from build123d import *

# Parameters (mm, degrees)
MODEL_R         = 24.25
MODEL_R_2       = 2
EXTRUDE_1_DEPTH = 2


with BuildPart() as part:
    # Model → 凸台-拉伸1 (new body)
    with BuildSketch(Plane.XY):
        with Locations((1461.027973693, 726.314415121)):
            Circle(MODEL_R)
        with Locations((1461.027973693, 726.314415121)):
            Circle(MODEL_R_2, mode=Mode.SUBTRACT)
        with BuildLine():
            ThreePointArc((1454.730507071, 746.347934885), (1450.527973693, 744.5009486), (1446.827169961, 741.784941077))
            ThreePointArc((1446.827169961, 741.784941077), (1445.858696219, 739.705372638), (1446.642743938, 737.549493362))
            ThreePointArc((1446.642743938, 737.549493362), (1449.919857233, 734.687570493), (1453.749968469, 732.623515752))
            ThreePointArc((1453.749968469, 732.623515752), (1457.242892618, 732.870367853), (1459.203134883, 735.771902849))
            ThreePointArc((1459.203134883, 735.771902849), (1459.33066666, 740.120903849), (1458.490725399, 744.389928648))
            ThreePointArc((1458.490725399, 744.389928648), (1457.015703038, 746.146873529), (1454.730507071, 746.347934885))
        make_face(mode=Mode.SUBTRACT)
        with BuildLine():
            ThreePointArc((1440.529703339, 730.877408929), (1440.027973693, 726.314415121), (1440.529703339, 721.751421313))
            ThreePointArc((1440.529703339, 721.751421313), (1441.846425564, 719.87291423), (1444.105495645, 719.473979835))
            ThreePointArc((1444.105495645, 719.473979835), (1448.222550201, 720.881081765), (1451.925129659, 723.166028024))
            ThreePointArc((1451.925129659, 723.166028024), (1453.457811542, 726.314415121), (1451.925129659, 729.462802217))
            ThreePointArc((1451.925129659, 729.462802217), (1448.222550201, 731.747748477), (1444.105495645, 733.154850407))
            ThreePointArc((1444.105495645, 733.154850407), (1441.846425564, 732.755916011), (1440.529703339, 730.877408929))
        make_face(mode=Mode.SUBTRACT)
        with BuildLine():
            ThreePointArc((1446.827169961, 710.843889164), (1450.527973693, 708.127881641), (1454.730507071, 706.280895356))
            ThreePointArc((1454.730507071, 706.280895356), (1457.015703038, 706.481956712), (1458.490725399, 708.238901593))
            ThreePointArc((1458.490725399, 708.238901593), (1459.33066666, 712.507926392), (1459.203134883, 716.856927392))
            ThreePointArc((1459.203134883, 716.856927392), (1457.242892618, 719.758462388), (1453.749968469, 720.005314489))
            ThreePointArc((1453.749968469, 720.005314489), (1449.919857233, 717.941259748), (1446.642743938, 715.079336879))
            ThreePointArc((1446.642743938, 715.079336879), (1445.858696219, 712.923457603), (1446.827169961, 710.843889164))
        make_face(mode=Mode.SUBTRACT)
        with BuildLine():
            ThreePointArc((1467.325440315, 706.280895356), (1471.527973693, 708.127881641), (1475.228777425, 710.843889164))
            ThreePointArc((1475.228777425, 710.843889164), (1476.197251167, 712.923457603), (1475.413203447, 715.079336879))
            ThreePointArc((1475.413203447, 715.079336879), (1472.136090152, 717.941259748), (1468.305978916, 720.005314489))
            ThreePointArc((1468.305978916, 720.005314489), (1464.813054768, 719.758462388), (1462.852812503, 716.856927392))
            ThreePointArc((1462.852812503, 716.856927392), (1462.725280725, 712.507926392), (1463.565221986, 708.238901593))
            ThreePointArc((1463.565221986, 708.238901593), (1465.040244347, 706.481956712), (1467.325440315, 706.280895356))
        make_face(mode=Mode.SUBTRACT)
        with BuildLine():
            ThreePointArc((1481.526244047, 721.751421313), (1482.027973693, 726.314415121), (1481.526244047, 730.877408929))
            ThreePointArc((1481.526244047, 730.877408929), (1480.209521821, 732.755916011), (1477.950451741, 733.154850407))
            ThreePointArc((1477.950451741, 733.154850407), (1473.833397185, 731.747748477), (1470.130817726, 729.462802217))
            ThreePointArc((1470.130817726, 729.462802217), (1468.598135843, 726.314415121), (1470.130817726, 723.166028024))
            ThreePointArc((1470.130817726, 723.166028024), (1473.833397185, 720.881081765), (1477.950451741, 719.473979835))
            ThreePointArc((1477.950451741, 719.473979835), (1480.209521821, 719.87291423), (1481.526244047, 721.751421313))
        make_face(mode=Mode.SUBTRACT)
        with BuildLine():
            ThreePointArc((1475.228777425, 741.784941077), (1471.527973693, 744.5009486), (1467.325440315, 746.347934885))
            ThreePointArc((1467.325440315, 746.347934885), (1465.040244347, 746.146873529), (1463.565221986, 744.389928648))
            ThreePointArc((1463.565221986, 744.389928648), (1462.725280725, 740.120903849), (1462.852812503, 735.771902849))
            ThreePointArc((1462.852812503, 735.771902849), (1464.813054768, 732.870367853), (1468.305978916, 732.623515752))
            ThreePointArc((1468.305978916, 732.623515752), (1472.136090152, 734.687570493), (1475.413203447, 737.549493362))
            ThreePointArc((1475.413203447, 737.549493362), (1476.197251167, 739.705372638), (1475.228777425, 741.784941077))
        make_face(mode=Mode.SUBTRACT)
    extrude(amount=EXTRUDE_1_DEPTH)


solid = part.part
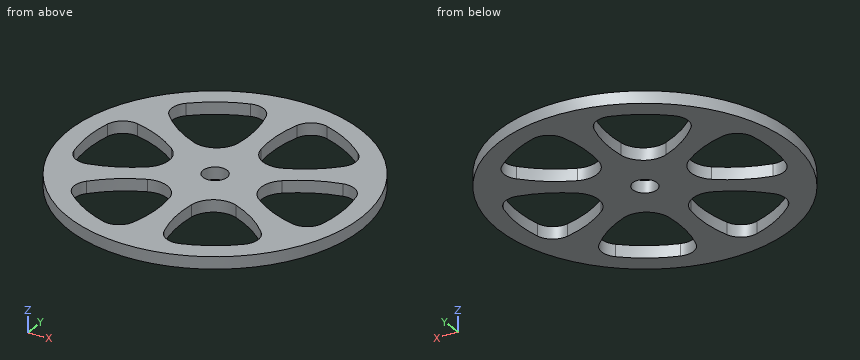
Source: CAD feature listing. Evaluate the final solid. Frame: model axes, mm. Round coordinates to 2 decimals unless told otherwise and drop trailing zeros. Loops run counter-clockwise (first coordinate to the right, second up) from the corner with the lowest first, then second, coordinate; pieces in that order, holes last. Notation, with made-up numbers: (13, -13) -> (31, -13) arc R16 ccw to (31, 15) -> close; hole circle Ø6 at (76, 74). An arc over 180 degrees is marked (long way). Answer as a JSON object with one key per item and string values. Group by question number.
Q1. Section query A-A (y = 737). Output: boundary loops of the cut face in (x, z), plus the area to 3 significant figures.
Q2. Ray query, line 1 (X direction, y = 725, z = 1.5); line 2 (Y direction, x = 1451.5, z = 1.55); line 3 (X direction, y = 739.5, z = 1.1). Return the intervals inside material, ascending. Write a range as from..to.
Q3. Section query D-D (y = 722.5). Output: boundary loops of the cut face in (x, z), plus the area to 3 significant figures.
Q4. Contact query for flat-ended pins moving along their axis: P1, Ø1, axis at x = 1474.5, z = 1, coming from the -Y side; P2, Ø1, axis at y = 709, z = 0.5, coming from the -X side. Output: stop coordinate, or through.
Q5. Section query C-C (x = 1479). Output: boundary loops of the cut face in (y, z).
Q6. Section query B-B (x = 1471). Output: boundary loops of the cut face in (y, z).
Completed:
{
 "1": {"outline": "(1439.26, 0) -> (1447.17, 0) -> (1447.17, 2) -> (1439.26, 2) -> close; (1459.34, 0) -> (1462.72, 0) -> (1462.72, 2) -> (1459.34, 2) -> close; (1474.89, 0) -> (1482.8, 0) -> (1482.8, 2) -> (1474.89, 2) -> close", "area": "38.4 mm²"},
 "2": {"line 1": "1436.81..1440.07, 1453.24..1459.52, 1462.54..1468.82, 1481.99..1485.24", "line 2": "704.01..707.6, 718.93..722.84, 729.79..733.7, 745.03..748.61", "line 3": "1440.68..1445.86, 1459.37..1462.68, 1476.2..1481.38"},
 "3": {"outline": "(1437.08, 0) -> (1440.38, 0) -> (1440.38, 2) -> (1437.08, 2) -> close; (1451.02, 0) -> (1471.03, 0) -> (1471.03, 2) -> (1451.02, 2) -> close; (1481.68, 0) -> (1484.98, 0) -> (1484.98, 2) -> (1481.68, 2) -> close", "area": "53.2 mm²"},
 "4": {"P1": "y = 705.83", "P2": "x = 1443.55"},
 "5": {"outline": "(710.03, 0) -> (719.43, 0) -> (719.43, 2) -> (710.03, 2) -> close; (733.2, 0) -> (742.6, 0) -> (742.6, 2) -> (733.2, 2) -> close"},
 "6": {"outline": "(704.21, 0) -> (707.83, 0) -> (707.83, 2) -> (704.21, 2) -> close; (718.67, 0) -> (722.52, 0) -> (722.52, 2) -> (718.67, 2) -> close; (730.11, 0) -> (733.96, 0) -> (733.96, 2) -> (730.11, 2) -> close; (744.8, 0) -> (748.42, 0) -> (748.42, 2) -> (744.8, 2) -> close"}
}
